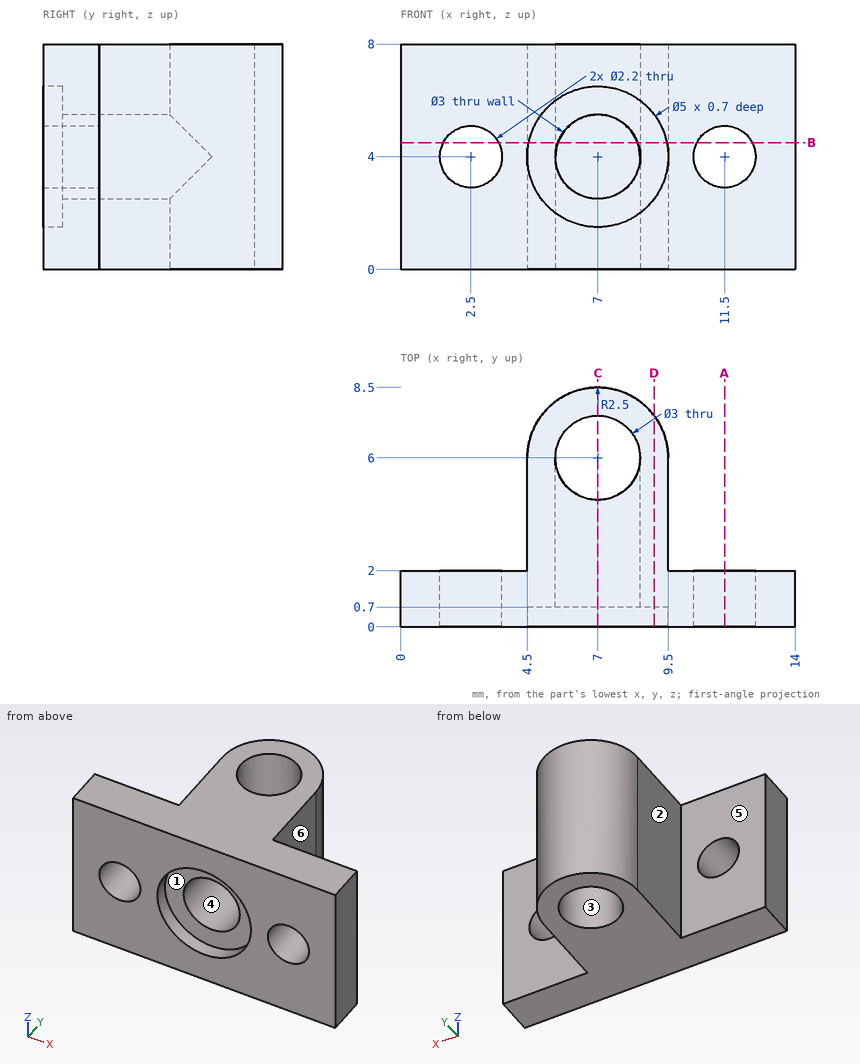
Drawing for the job (mm, zero at the part's lowest x, y, z). A direction names the side the tool comes from. Give positions to 0.01 mm unless a question says otherwise; leave off trailing zeros. Order: outer loops, then holes, each group sorted by start corner. A loop starts at its lowest first (then second) coordinate and runs counter-clockwise, first axis right, second up. Notation, with made-up numbers: M 56,29.5 L 73,29.5 A33 cw 73,68.5 Z; hole C 45,42 d9. An arc over 180 degrees is marked long. Use a Markdown table: item, result. Add a question column.
(1) Saw through at C-C, the plane x = 7. Give the cut face in (y, z), and give its area (3 significant figures).
(2) Saw through at A-A, the plane x = 11.5. Give the cut face in (y, z), and give its area (3 significant figures).
(3) Saw through at B-B, the plane z = 4.5. Give the cut face in (x, y), and give its area (3 significant figures).
(4) Probe line 1 along X through (y, z) = (0.45, 4); line 2 along X through (y, z) = (0.5, 3); line 3 along Z through (x, y) = (7, 2.75). List the from-to ranges inside material, lowest first. Write a range as [from, to].
(5) Saw through at D-D, the plane x = 9. Give the cut face in (y, z), and give its area (3 significant figures).
(6) Mould opens along Y. For the marked faces 1, 2 and 3 say: +Y half, -Y half, draft (parallel to the pull), parting line (faces both ways), or undercut.
(7) 3-axis set-ups, long thin cutter, end or side, ignore diameter. For the marked faces 4, 5 and 6: which of +Z, -Z, +X, -X, +Y, -Y reach the whole face in a straight line?
(8) Drop flat-ended pins along their axis: P1, Ø1.2, axis at y = 5, z = 4, coming from the +X side; P2, Ø1.8, axis at x = 11.5, z = 4, coming from the -Y side; P3, Ø1.3, axis at x = 1.5, z = 4, coming from the +Y side; P4, Ø1.2, axis at y = 3.5, z = 3.5, coming from the -X side. Give the stop position or say it passes through.
Answer key:
| question | item | result |
|---|---|---|
| 1 | outline | M 0,0 L 4.5,0 L 4.5,2.5 L 0.7,2.5 L 0.7,1.5 L 0,1.5 Z; M 0,6.5 L 0.7,6.5 L 0.7,5.5 L 4.5,5.5 L 4.5,8 L 0,8 Z; M 7.5,0 L 8.5,0 L 8.5,8 L 7.5,8 Z |
| 1 | area | 29.1 mm^2 |
| 2 | outline | M 0,0 L 2,0 L 2,2.9 L 0,2.9 Z; M 0,5.1 L 2,5.1 L 2,8 L 0,8 Z |
| 2 | area | 11.6 mm^2 |
| 3 | outline | M 0,0 L 1.52,0 L 1.52,2 L 0,2 Z; M 3.48,0 L 4.55,0 L 4.55,0.7 L 5.59,0.7 L 5.59,5.5 A1.5 cw long 8.41,5.5 L 8.41,0.7 L 9.45,0.7 L 9.45,0 L 10.52,0 L 10.52,2 L 9.5,2 L 9.5,6 A2.5 ccw 4.5,6 L 4.5,2 L 3.48,2 Z; M 12.48,0 L 14,0 L 14,2 L 12.48,2 Z |
| 3 | area | 28.0 mm^2 |
| 4 | line 1 | [0, 1.4], [3.6, 4.5], [9.5, 10.4], [12.6, 14] |
| 4 | line 2 | [0, 2.04], [2.96, 4.71], [9.29, 11.04], [11.96, 14] |
| 4 | line 3 | [0, 2.5], [5.5, 8] |
| 5 | outline | M 0,0 L 7.5,0 L 7.5,8 L 0,8 L 0,5.5 L 0.7,5.5 L 0.7,2.5 L 0,2.5 Z |
| 5 | area | 57.9 mm^2 |
| 6 | face 1 | -Y half |
| 6 | face 2 | draft |
| 6 | face 3 | undercut |
| 7 | face 4 | -Y |
| 7 | face 5 | +Z, -Z, -X, +Y |
| 7 | face 6 | +Z, -Z, +X, +Y |
| 8 | P1 | x = 9.5 |
| 8 | P2 | through |
| 8 | P3 | y = 2 |
| 8 | P4 | x = 4.5 |
